Part model, mm, in its own coordinate system. A direction names the side the tool comes from. Round coordinates to 2 decimals unless told otherwise and drop trailing zeros. Loops run counter-clockwise (first coordinate to the right, second up) from the corner with the lowest first, then second, coordinate; pieces in that order, holes last. Notation, with made-up numbers: (83, 8.5) -> (140, 8.5) arc R9 ccw to (140, 23.5) -> close; hole circle Ø7 at (-2, 77). An arc over 180 degrees is marked (long way). Answer as CSV lines item,"result".
from build123d import *

# Parameters (mm, degrees)
SKETCH1_R           = 1.5875
BOSS_EXTRUDE1_DEPTH = 3.175


with BuildPart() as part:
    # Sketch1 → Boss-Extrude1 (new body)
    with BuildSketch(Plane(origin=(0, 0, 0), x_dir=(1, 0, 0), z_dir=(0, 1, 0))):
        with BuildLine():
            ThreePointArc((-1.625434965, 4.675517209), (-2.013346383, 4.522050015), (-2.386958137, 4.336465249))
            ThreePointArc((-2.386958137, 4.336465249), (-2.952961664, 5.077251852), (-3.758538597, 5.546475243))
            ThreePointArc((-3.758538597, 5.546475243), (-3.93816119, 5.420413862), (-4.113559122, 5.288537733))
            ThreePointArc((-4.113559122, 5.288537733), (-3.916238121, 4.37739054), (-3.386612903, 3.610173548))
            ThreePointArc((-3.386612903, 3.610173548), (-3.678566886, 3.312196501), (-3.944394082, 2.99069479))
            ThreePointArc((-3.944394082, 2.99069479), (-4.762769089, 3.437222652), (-5.689550583, 3.538221892))
            ThreePointArc((-5.689550583, 3.538221892), (-5.802370205, 3.35), (-5.908965335, 3.158184395))
            ThreePointArc((-5.908965335, 3.158184395), (-5.35810668, 2.406067698), (-4.562214704, 1.920598082))
            ThreePointArc((-4.562214704, 1.920598082), (-4.707729756, 1.529634122), (-4.819808456, 1.127806033))
            ThreePointArc((-4.819808456, 1.127806033), (-5.74905047, 1.20286643), (-6.636787586, 0.918177833))
            ThreePointArc((-6.636787586, 0.918177833), (-6.663296699, 0.700340704), (-6.68265776, 0.481752285))
            ThreePointArc((-6.68265776, 0.481752285), (-5.873509917, 0.018713892), (-4.948968136, -0.10106624))
            ThreePointArc((-4.948968136, -0.10106624), (-4.922883382, -0.517415893), (-4.861834162, -0.930090633))
            ThreePointArc((-4.861834162, -0.930090633), (-5.741268797, -1.239476326), (-6.436463722, -1.860627515))
            ThreePointArc((-6.436463722, -1.860627515), (-6.372078659, -2.070413862), (-6.300857949, -2.277979173))
            ThreePointArc((-6.300857949, -2.277979173), (-5.373329931, -2.371875716), (-4.480000018, -2.105255291))
            ThreePointArc((-4.480000018, -2.105255291), (-4.286825749, -2.475), (-4.063204572, -2.827166179))
            ThreePointArc((-4.063204572, -2.827166179), (-4.74076959, -3.467502365), (-5.123216807, -4.317713463))
            ThreePointArc((-5.123216807, -4.317713463), (-4.979070331, -4.483175063), (-4.829582556, -4.643827336))
            ThreePointArc((-4.829582556, -4.643827336), (-3.944052384, -4.352346465), (-3.236399197, -3.745426576))
            ThreePointArc((-3.236399197, -3.745426576), (-2.909536999, -4.004634122), (-2.562009999, -4.235399009))
            ThreePointArc((-2.562009999, -4.235399009), (-2.920548253, -5.095965744), (-2.924119163, -6.028227527))
            ThreePointArc((-2.924119163, -6.028227527), (-2.725135509, -6.120754566), (-2.523228465, -6.206715566))
            ThreePointArc((-2.523228465, -6.206715566), (-1.83281235, -5.58025697), (-1.433195553, -4.737979581))
            ThreePointArc((-1.433195553, -4.737979581), (-1.02916287, -4.841830624), (-0.617820622, -4.911292872))
            ThreePointArc((-0.617820622, -4.911292872), (-0.595337591, -5.84329035), (-0.219414751, -6.696406287))
            ThreePointArc((-0.219414751, -6.696406287), (0, -6.7), (0.219414751, -6.696406287))
            ThreePointArc((0.219414751, -6.696406287), (0.595337591, -5.84329035), (0.617820622, -4.911292872))
            ThreePointArc((0.617820622, -4.911292872), (1.02916287, -4.841830624), (1.433195553, -4.737979581))
            ThreePointArc((1.433195553, -4.737979581), (1.83281235, -5.58025697), (2.523228465, -6.206715566))
            ThreePointArc((2.523228465, -6.206715566), (2.725135509, -6.120754566), (2.924119163, -6.028227527))
            ThreePointArc((2.924119163, -6.028227527), (2.920548253, -5.095965744), (2.562009999, -4.235399009))
            ThreePointArc((2.562009999, -4.235399009), (2.909536999, -4.004634122), (3.236399197, -3.745426576))
            ThreePointArc((3.236399197, -3.745426576), (3.944052384, -4.352346465), (4.829582556, -4.643827336))
            ThreePointArc((4.829582556, -4.643827336), (4.979070331, -4.483175063), (5.123216807, -4.317713463))
            ThreePointArc((5.123216807, -4.317713463), (4.74076959, -3.467502365), (4.063204572, -2.827166179))
            ThreePointArc((4.063204572, -2.827166179), (4.286825749, -2.475), (4.480000018, -2.105255291))
            ThreePointArc((4.480000018, -2.105255291), (5.373329931, -2.371875716), (6.300857949, -2.277979173))
            ThreePointArc((6.300857949, -2.277979173), (6.372078659, -2.070413862), (6.436463722, -1.860627515))
            ThreePointArc((6.436463722, -1.860627515), (5.741268797, -1.239476326), (4.861834162, -0.930090633))
            ThreePointArc((4.861834162, -0.930090633), (4.922883382, -0.517415893), (4.948968136, -0.10106624))
            ThreePointArc((4.948968136, -0.10106624), (5.873509917, 0.018713892), (6.68265776, 0.481752285))
            ThreePointArc((6.68265776, 0.481752285), (6.663296699, 0.700340704), (6.636787586, 0.918177833))
            ThreePointArc((6.636787586, 0.918177833), (5.74905047, 1.20286643), (4.819808456, 1.127806033))
            ThreePointArc((4.819808456, 1.127806033), (4.707729756, 1.529634122), (4.562214704, 1.920598082))
            ThreePointArc((4.562214704, 1.920598082), (5.35810668, 2.406067698), (5.908965335, 3.158184395))
            ThreePointArc((5.908965335, 3.158184395), (5.802370205, 3.35), (5.689550583, 3.538221892))
            ThreePointArc((5.689550583, 3.538221892), (4.762769089, 3.437222652), (3.944394082, 2.99069479))
            ThreePointArc((3.944394082, 2.99069479), (3.678566886, 3.312196501), (3.386612903, 3.610173548))
            ThreePointArc((3.386612903, 3.610173548), (3.916238121, 4.37739054), (4.113559122, 5.288537733))
            ThreePointArc((4.113559122, 5.288537733), (3.93816119, 5.420413862), (3.758538597, 5.546475243))
            ThreePointArc((3.758538597, 5.546475243), (2.952961664, 5.077251852), (2.386958137, 4.336465249))
            ThreePointArc((2.386958137, 4.336465249), (2.013346383, 4.522050015), (1.625434965, 4.675517209))
            ThreePointArc((1.625434965, 4.675517209), (1.797216412, 5.591822791), (1.606881166, 6.504454852))
            ThreePointArc((1.606881166, 6.504454852), (1.393008328, 6.553588925), (1.177641141, 6.595692636))
            ThreePointArc((1.177641141, 6.595692636), (0.632560341, 5.839378081), (0.416795446, 4.93242147))
            ThreePointArc((0.416795446, 4.93242147), (0, 4.95), (-0.416795446, 4.93242147))
            ThreePointArc((-0.416795446, 4.93242147), (-0.632560341, 5.839378081), (-1.177641141, 6.595692636))
            ThreePointArc((-1.177641141, 6.595692636), (-1.393008328, 6.553588925), (-1.606881166, 6.504454852))
            ThreePointArc((-1.606881166, 6.504454852), (-1.797216412, 5.591822791), (-1.625434965, 4.675517209))
        make_face()
        Circle(SKETCH1_R, mode=Mode.SUBTRACT)
    extrude(amount=BOSS_EXTRUDE1_DEPTH)


solid = part.part
Q1. Saw through at B-B, the plane z = 0.75. Write the cut outline in (x, y) (3 decimals), then the cut area to 3 significant figures.
Geometry results:
outline,"(-4.893, 0) -> (-1.399, 0) -> (-1.399, 3.175) -> (-4.893, 3.175) -> close; (1.399, 0) -> (4.893, 0) -> (4.893, 3.175) -> (1.399, 3.175) -> close"
area,"22.2 mm2"
Q2. Drop a flat-ended pin along its axis: P1, Ø1, axis at y = 1.5, z = 1.5, coming from the +X side. Give the stop position or say it passes through.
Geometry results:
P1,"x = 6.44"
Q3. Drill centre lines: line 1 along Z through (x, y) = (0, 0.8); line 2 along Z through (x, y) = (1, 0.8); line 3 along X through (y, z) = (1.25, -0.75). Where is each one in solid material? Low to high.
Geometry results:
line 1,"-4.95 to -1.59, 1.59 to 6.7"
line 2,"-6.41 to -1.23, 1.23 to 4.85"
line 3,"-6.66 to -1.4, 1.4 to 6.66"
Q4. Two-plate mould, pull along X, no slides. Class faces 6 (the face through (0.638, 1.565, -5.851)), 7 (the face through (1, 0, -2)), 8 (the face through (5.35, 1.57, -2.4)): pulls with the +X half, pulls with the -X half, needs draft (parallel to the pull), parting line crosses it, or undercut.
Geometry results:
face 6,"undercut"
face 7,"needs draft"
face 8,"pulls with the +X half"
Q5. Which spindle directions (+Z, -Z, +X, -X, +Y, -Y) get a long thin tool onto all of the face, cutting with end or side? Do faces 1 (the face through (-5.73, 1.565, 1.233)), 2 (the face through (-2.918, 1.565, 5.083)), 3 (the face through (4.75, 1.57, 3.48)), 4 (the face through (-0.63, 1.57, -5.83)), 5 (the face through (1.825, 1.565, 5.57)). Say none if no direction does.
Geometry results:
face 1,"-X, +Y, -Y"
face 2,"+Y, -Y"
face 3,"+X, +Y, -Y"
face 4,"-Z, +Y, -Y"
face 5,"+Z, +Y, -Y"
Q6. Saw through at C-C, the plane x = 5.5. Write the cut outline in (y, z) (3 decimals), then the cut area to 3 significant figures.
Geometry results:
outline,"(0, -3.547) -> (3.175, -3.547) -> (3.175, -2.548) -> (0, -2.548) -> close; (0, -1.219) -> (3.175, -1.219) -> (3.175, 0.074) -> (0, 0.074) -> close; (0, 1.115) -> (3.175, 1.115) -> (3.175, 2.381) -> (0, 2.381) -> close"
area,"11.3 mm2"
